Job drawing, mm, ordinate dimensions from the low corner. One solid piece. Round coordinates to 2 decimals unless told otherwise and drop trailing zeros. Loops run counter-clockwise (first coordinate to the right, second up) from the corner with the lowest first, then second, coordinate; pieces in that order, holes last.
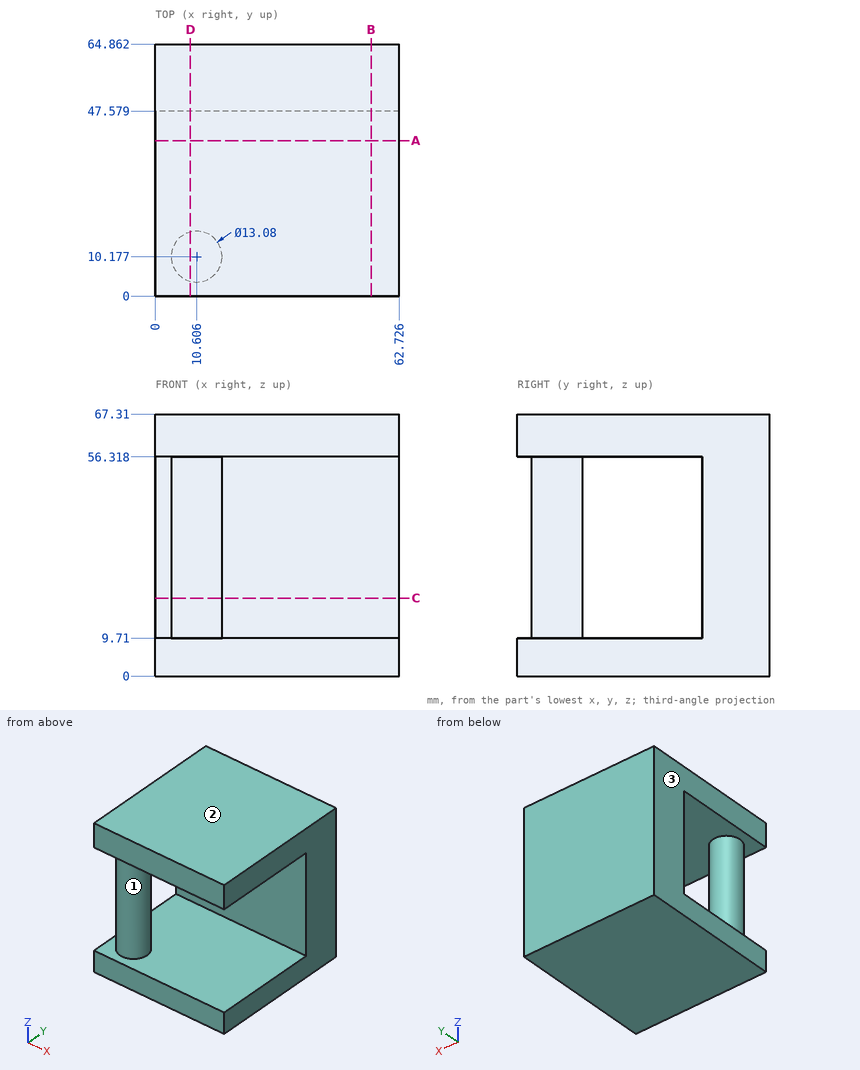
Item 1: Probe line 1 (Z direction, x = 54.5, y = 44.5); line 2 (Y direction, x = 39, z = 33.5); line 3 (Y direction, x = 7, z = 39.5) (1 decimal). List the from-to ranges inside material, lowest first.
Answers follow:
line 1: z = 0 to 9.71, 56.32 to 67.31
line 2: y = 47.58 to 64.86
line 3: y = 4.7 to 15.6, 47.6 to 64.9
Item 2: Two-plate mould, pull along Z, no slides. Class the marked faces 1, 2 and 3: released by +Z, released by -Z, zero draft, split by the parting line, or undercut.
Answers follow:
face 1: undercut
face 2: released by +Z
face 3: zero draft
Item 3: Cut at B-B, the plane x = 55.5. Give the cut face in (y, z).
Answers follow:
outline: (0, 0) - (64.86, 0) - (64.86, 67.31) - (0, 67.31) - (0, 56.32) - (47.58, 56.32) - (47.58, 9.71) - (0, 9.71) - close
Item 4: Cut at D-D, the plane x = 9. Give the cut face in (y, z), plus the area to 3 significant figures.
Answers follow:
outline: (0, 0) - (64.86, 0) - (64.86, 67.31) - (0, 67.31) - (0, 56.32) - (3.84, 56.32) - (3.84, 9.71) - (0, 9.71) - close; hole (16.52, 9.71) - (47.58, 9.71) - (47.58, 56.32) - (16.52, 56.32) - close
area: 2,740 mm2
Item 5: Cut at A-A, the plane y = 40. Give the cut face in (x, z).
Answers follow:
outline: (0, 0) - (62.73, 0) - (62.73, 9.71) - (0, 9.71) - close; (0, 56.32) - (62.73, 56.32) - (62.73, 67.31) - (0, 67.31) - close
Item 6: Flat gauge pin, fed straight in: P1, Ø23.5, axis at x = 46.5, z = 30.5, coming from the -Y side. Where does the tip first touch, or does it go through?
Answers follow:
P1: stops at y = 47.58
Item 7: Cut at C-C, the plane z = 20. Give the cut face in (x, y) (1 decimal).
Answers follow:
outline: (0, 47.6) - (62.7, 47.6) - (62.7, 64.9) - (0, 64.9) - close; circle Ø13.1 at (10.6, 10.2)
